Autodesk Inventor part; units mm, degrees
ref_plane "YZ Plane" through (0, 0, 0) normal (1, 0, 0) x (0, 1, 0)
ref_plane "XZ Plane" through (0, 0, 0) normal (0, 1, 0) x (-1, 0, 0)
ref_plane "XY Plane" through (0, 0, 0) normal (0, 0, 1) x (1, 0, 0)
sketch "Sketch1" plane through (0, 0, 0) normal (0, 1, 0) x (-1, 0, 0)
  line L0 (-50, 50) -> (50, 50)
  line L1 (50, 50) -> (50, -50)
  line L2 (50, -50) -> (-50, -50)
  line L3 (-50, -50) -> (-50, 50)
  line L4 (-50, 50) -> (50, -50) construction
  line L5 (50, 50) -> (-50, -50) construction
  point P0 (0, 0)
  dimension "d0" = 100
sketch "Sketch2" plane through (0, 0, 0) normal (0, 0, 1) x (1, 0, 0)
  line L0 (0, -6.18) -> (0, 36.03)
  line L1 (50, 0) -> (-50, 0)
  line L2 (-45, 0) -> (0, 30) construction
  line L3 (0, 30) -> (45, 0) construction
  spline S0 degree 2 poles (-45, 0) (0, 30) (45, 0) knots 1 1 1 2 2 2
  point P0 (0, 0)
  point P1 (0, 0)
  point P2 (0, 15)
  dimension "d1" = 30
  dimension "d2" = 5
extrude "Extrusion1" add sketch "Sketch1" against normal blind 10
revolve "Revolution2" add sketch "Sketch2" angle 360 about axis through (0, -10, 0) along (0, 1, 0) picked at (-26.1787, 2.223) contours L1 S0 L0
fillet "Fillet1" radius 5 1 edges at (45, 0, 0)
properties part number "Surface1"
The model under review builds one solid part; all positions refer to its coordinate system, in mm. A direction names the side the tool comes from. Round coordinates to 2 decimals unless told otherwise and drop trailing zeros. Write item = value, one per line. Start each with the question number.
Item 1: For faces 1 (the flat face through (45.1, 0, 12.3)), 2 (the flat face through (-50, -5, 1)), list the 3-axis set-ups (+Z, -Z, +X, -X, +Y, -Y) from which the entire face can be reached by the end or side of a thin tool; tool diameter is ignored.
Item 2: Insertion check: pin 1 (8 mm diameter, centred on x = 0.5, y = 7, fed in from +Z); pin 2 (1 mm diameter, centred on x = -20, z = -2.5, fed in from +Y). Each pin has a flat end and moves straight along its axis. Give the tip position at first contact, or say it passes through.
Item 3: To check wall thickness, follow L1, parallel to Y at x = 34.5, z = -39.5; L2, parallel to Y at x = -37.5, z = 6.5; L3, parallel to Z at x = -8, y = 2.75. State the ranges of each line that lie inside material, in increasing order.
Result:
q1.face_1 = +Y
q1.face_2 = +Z, -Z, -X, +Y, -Y
q2.pin_1 = 40.25
q2.pin_2 = 12.14
q3.L1 = -10 to 0
q3.L2 = -10 to 4.27
q3.L3 = -39.87 to 39.87
